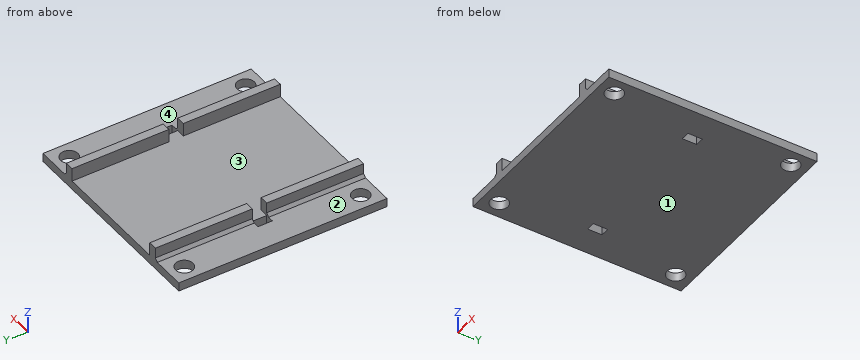
from build123d import *

# Parameters (mm, degrees)
F0_W     = 6.2
F0_H     = 36
F0_R     = 1.5
F0_W_2   = 1.5
F0_W_3   = 20.6
F3_DEPTH = 1.5
F4_DEPTH = 3.8
F2_W     = 1.5
F2_H     = 2.5
F5_DEPTH = 25
F6_SIZE  = 0.5
F7_W     = 1.5
F7_H     = 2.5
F8_DEPTH = 25


with BuildPart() as f3:
    # F0 (on Top) → F3 (new body)
    with BuildSketch(Plane.XY):
        with Locations((14.9, 0)):
            Rectangle(F0_W, F0_H)
        with Locations((15.25, -15.25)):
            Circle(F0_R, mode=Mode.SUBTRACT)
        with Locations((15.25, 15.25)):
            Circle(F0_R, mode=Mode.SUBTRACT)
        with Locations((11.05, 0)):
            Rectangle(F0_W_2, F0_H)
        Rectangle(F0_W_3, F0_H)
        with Locations((-11.05, 0)):
            Rectangle(F0_W_2, F0_H)
        with Locations((-14.9, 0)):
            Rectangle(F0_W, F0_H)
        with Locations((-15.25, -15.25)):
            Circle(F0_R, mode=Mode.SUBTRACT)
        with Locations((-15.25, 15.25)):
            Circle(F0_R, mode=Mode.SUBTRACT)
    extrude(amount=F3_DEPTH)

    # F0 (on Top) → F4 (join)
    with BuildSketch(Plane.XY):
        with Locations((-11.05, 0)):
            Rectangle(F0_W_2, F0_H)
        with Locations((11.05, 0)):
            Rectangle(F0_W_2, F0_H)
    extrude(amount=F4_DEPTH)

    # F2 (on face) → F5 (cut)
    with BuildSketch(Plane.XY):
        with Locations((-12.55, 0)):
            Rectangle(F2_W, F2_H)
        with Locations((12.55, 0)):
            Rectangle(F2_W, F2_H)
    extrude(amount=F5_DEPTH, mode=Mode.SUBTRACT)

    # F6
    f6_edges = [f3.edges().sort_by_distance(p)[0] for p in [
        (-11.8, 9.625, 1.5),
        (-11.8, -9.625, 1.5),
        (11.8, -9.625, 1.5),
        (11.8, 9.625, 1.5),
    ]]
    chamfer(f6_edges, length=F6_SIZE)

    # F7 (on face) → F8 (cut)
    with BuildSketch(Plane.XY.offset(1.5)):
        with Locations((-11.05, 0)):
            Rectangle(F7_W, F7_H)
        with Locations((11.05, 0)):
            Rectangle(F7_W, F7_H)
    extrude(amount=F8_DEPTH, mode=Mode.SUBTRACT)


solid = f3.part
Could you check a few things on this model? Use its own coordinates, in mm. Face numbers are marked on the shaded views. A direction names the side the tool comes from. Coordinates: 2 decimals unless noted, no trailing zeros. Order: outer loops, then holes, each group sorted by start corner. A loop starts at its lowest first (then second) coordinate and runs counter-clockwise, first axis right, second up. Notation, with made-up numbers: (68.25, 0.5) - (94.25, 0.5) arc R28 cw to (94.25, 23.5) - close; hole circle Ø9 at (-12.5, -17). An arc over 180 degrees is marked (long way). Answer in a Markdown table with one row per item. Add a question column.
(1) Will these pins go through, and if not, where does the flat tip stop? pin 1 (0.9 mm diameter, centred on y = 13, z = 2.5, fed in from -X); pin 2 (5 mm diameter, centred on x = 3, y = 3, fed in from +Z); pin 3 (1.8 mm diameter, centred on y = -5.5, z = 3, fed in from +X); pin 4 (6 mm diameter, centred on x = 10, y = -3, fed in from +Z).
(2) If we section it at C-C, the plane z = 3.3: Please give me the cut outline in (x, y).
(3) If we section it at A-A, the plane z = 0.7: Please give me the cut outline in (x, y).
(4) On a 3-axis mill with a long thin cutter (end or side, diameter ignored), from which of +Z, -Z, +X, -X, +Y, -Y can I reach the whole of each face in a straight line? I mean the marked faces 1 and 2. Say none if no direction works.
(5) I need wall thicknesses on L1, parallel to Y at x = -15.25, z = 1; L2, parallel to X at y = 16.5, z = 0.9; L3, parallel to X at y = -6, z = 3.5. Which ranges of each line are inside material? Lowest first, please.
(6) If we section it at D-D, the plane y = -15.25: Please give me the cut outline in (x, z).
(7) If we mould it in two halves opening along X, with no side actions, what happens to the marked faces 3 and 4? For each: released by +X, released by -X, zero draft, split by the parting line, or undercut.
(8) If we section it at B-B, the plane x = -15.25: Please give me the cut outline in (y, z), then the cut area to 3 significant figures.
Results are:
| question | item | result |
|---|---|---|
| 1 | pin 1 | stops at x = -11.8 |
| 1 | pin 2 | stops at z = 1.5 |
| 1 | pin 3 | stops at x = 11.8 |
| 1 | pin 4 | stops at z = 3.8 |
| 2 | outline | (-11.8, -18) - (-10.3, -18) - (-10.3, -1.25) - (-11.8, -1.25) - close; (-11.8, 1.25) - (-10.3, 1.25) - (-10.3, 18) - (-11.8, 18) - close; (10.3, -18) - (11.8, -18) - (11.8, -1.25) - (10.3, -1.25) - close; (10.3, 1.25) - (11.8, 1.25) - (11.8, 18) - (10.3, 18) - close |
| 3 | outline | (-18, -18) - (18, -18) - (18, 18) - (-18, 18) - close; hole circle Ø3 at (-15.25, -15.25); hole circle Ø3 at (-15.25, 15.25); hole (-13.3, -1.25) - (-11.8, -1.25) - (-11.8, 1.25) - (-13.3, 1.25) - close; hole (11.8, -1.25) - (13.3, -1.25) - (13.3, 1.25) - (11.8, 1.25) - close; hole circle Ø3 at (15.25, -15.25); hole circle Ø3 at (15.25, 15.25) |
| 4 | face 1 | -Z, +X, -X, +Y, -Y |
| 4 | face 2 | +Z, -X, +Y, -Y |
| 5 | L1 | y = -18 to -16.75, -13.75 to 13.75, 16.75 to 18 |
| 5 | L2 | x = -18 to -16.08, -14.42 to 14.42, 16.08 to 18 |
| 5 | L3 | x = -11.8 to -10.3, 10.3 to 11.8 |
| 6 | outline | (-18, 0) - (-16.75, 0) - (-16.75, 1.5) - (-18, 1.5) - close; (-13.75, 0) - (13.75, 0) - (13.75, 1.5) - (12.3, 1.5) - (11.8, 2) - (11.8, 3.8) - (10.3, 3.8) - (10.3, 1.5) - (-10.3, 1.5) - (-10.3, 3.8) - (-11.8, 3.8) - (-11.8, 2) - (-12.3, 1.5) - (-13.75, 1.5) - close; (16.75, 0) - (18, 0) - (18, 1.5) - (16.75, 1.5) - close |
| 7 | face 3 | undercut |
| 7 | face 4 | zero draft |
| 8 | outline | (-18, 0) - (-16.75, 0) - (-16.75, 1.5) - (-18, 1.5) - close; (-13.75, 0) - (13.75, 0) - (13.75, 1.5) - (-13.75, 1.5) - close; (16.75, 0) - (18, 0) - (18, 1.5) - (16.75, 1.5) - close |
| 8 | area | 45.0 mm2 |
